Geometry check sheet. Reference: drawing and pictorial views, mm from the part's lowest x, y, z. Coordinates: 2 decimals unless noted, no trailing zeros. Loops run counter-clockwise (first coordinate to the right, second up) from the corner with the lowest first, then second, coordinate; pieces in that order, holes last. Notation, with made-up numbers: M 22.5,56 L 42.5,56 A13 ccw 42.5,69 Z; hole C 56.25,21 d6. An arc over 180 degrees is marked long. Write each question's results on one line, items separated by ' | '. Start each with the question number.
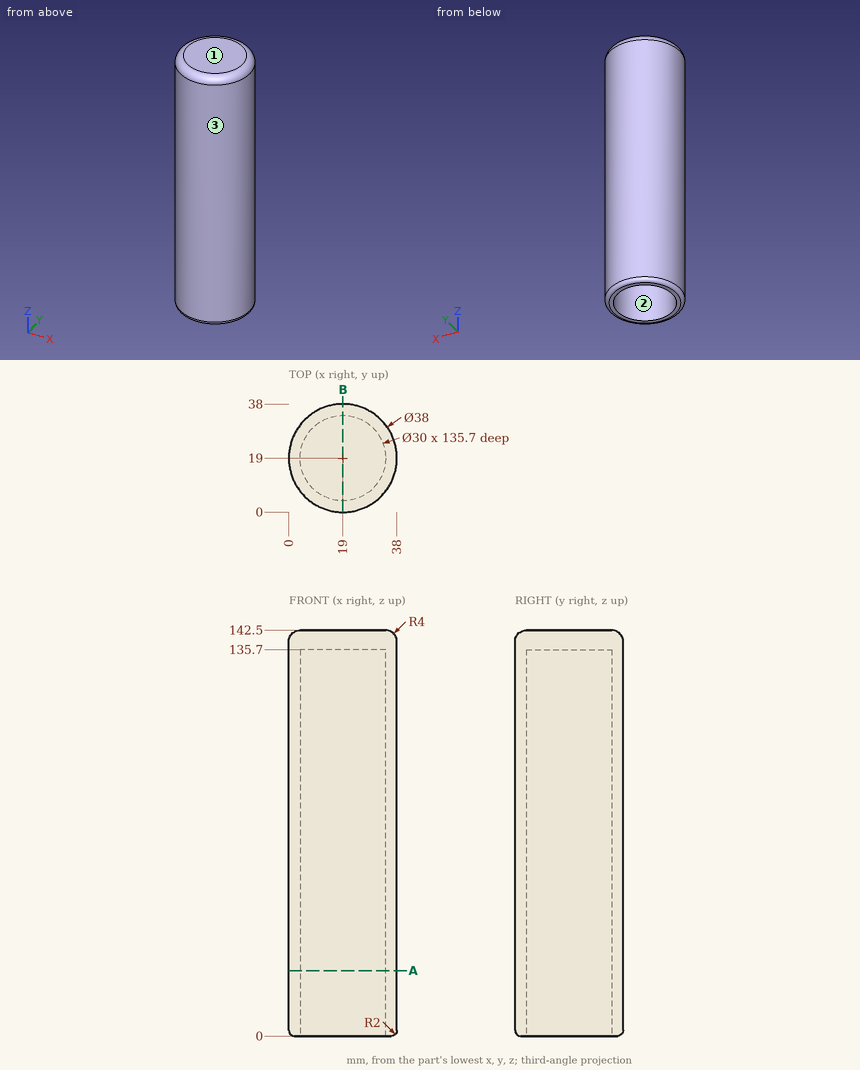
1) Release check for a two-part mould opening along X. For the marked faces 1, 2 and 3 record: +X half, -X half, draft (parallel to the pull), parting line (faces both ways), or undercut.
2) Section check B-B (x = 19). Enter the section's corners in (y, z), then the cut area to 3 significant figures.
3) Thickness scan on probe 1 along Y at (x, z) = (19, 108); probe 2 along X at (y, z) = (22.5, 102.5); probe 3 along Z at (x, y) = (17, 32). Record the ranges inside material, lowest first.
4) Gauge pin test, flat ends, axial feed: P1, Ø5, axis at x = 31.5, y = 29.5, coming from the +Z side; P2, Ø2, axis at y = 12.5, z = 64.5, coming from the -X side; P3, Ø1.5, axis at x = 32, z = 16, coming from the +Y side; P4, Ø1.5, axis at y = 23, z = 48, coming from the -X side. Record the tip position at first contact, or that the pin passes through.
5) Section check A-A (z = 23). Enter the section's corners in (x, y).
Return value:
1) face 1: draft | face 2: undercut | face 3: parting line
2) outline: M 0,2 A2 ccw 2,0 L 4,0 L 4,135.7 L 34,135.7 L 34,0 L 36,0 A2 ccw 38,2 L 38,138.5 A4 ccw 34,142.5 L 4,142.5 A4 ccw 0,138.5 Z | area: 1,340 mm2
3) probe 1: y = 0 to 4, 34 to 38 | probe 2: x = 0.33 to 4.41, 33.59 to 37.67 | probe 3: z = 135.7 to 142.5
4) P1: stops at z = 142.5 | P2: stops at x = 0.81 | P3: stops at y = 33.52 | P4: stops at x = 0.28
5) outline: C 19,19 d38; hole C 19,19 d30
